Design review of the part built by this model. Coordinates are the model's own, in mm. A direction names the side the tool comes from. Round coordinates to 2 decimals unless told otherwise and drop trailing zeros. Order: outer loops, then holes, each group sorted by start corner. A loop starts at its lowest first (then second) coordinate and runs counter-clockwise, first axis right, second up. Notation, with made-up numbers: (7, -21) - (16, -21) arc R12 ccw to (16, -2) - close; hole circle Ø10 at (54.5, 77). An arc over 180 degrees is marked (long way). Answer as a JSON object with one key per item and string values. Group by question number.
from build123d import *

# Parameters (mm, degrees)
EXTRUDE_1_DEPTH     = 50
SKETCH_2_W          = 4
SKETCH_2_H          = 24
EXTRUDE_2_DEPTH     = 210
CUT_EXTRUDE_1_DEPTH = 93
SKETCH_4_W          = 4
SKETCH_4_H          = 24
EXTRUDE_3_DEPTH     = 260
EXTRUDE_4_DEPTH     = 30
SKETCH_6_R          = 4
CUT_EXTRUDE_2_DEPTH = 97
SKETCH_8_W          = 162.90282803
SKETCH_8_H          = 303.086270548
CUT_EXTRUDE_4_DEPTH = 86
EXTRUDE_5_DEPTH     = 40
SKETCH_10_R         = 10
EXTRUDE_6_DEPTH     = 80


with BuildPart() as part:
    # 草图1 → 凸台-拉伸1 (new body, symmetric)
    with BuildSketch(Plane(origin=(0, 0, 0), x_dir=(1, 0, 0), z_dir=(0, 1, 0))):
        with BuildLine():
            Line((-46, 0), (-46, 12))
            Line((-46, 12), (-42, 12))
            Line((-42, 12), (-42, 0))
            ThreePointArc((-42, 0), (0, -42), (42, 0))
            Line((42, 0), (42, 12))
            Line((42, 12), (46, 12))
            Line((46, 12), (46, 0))
            ThreePointArc((46, 0), (37.456641601, -26.702059846), (15, -43.48562981))
            Line((15, -43.48562981), (15, -73))
            Line((15, -73), (10, -73))
            Line((10, -73), (10, -53))
            Line((10, -53), (-10, -53))
            Line((-10, -53), (-10, -73))
            Line((-10, -73), (-15, -73))
            Line((-15, -73), (-15, -43.48562981))
            ThreePointArc((-15, -43.48562981), (-37.456641601, -26.702059846), (-46, 0))
        make_face()
    extrude(amount=EXTRUDE_1_DEPTH, both=True)

    # 草图2 → 凸台-拉伸2 (add)
    with BuildSketch(Plane(origin=(0, 50, 0), x_dir=(1, 0, 0), z_dir=(0, 1, 0))):
        with Locations((-44, 0)):
            Rectangle(SKETCH_2_W, SKETCH_2_H)
        with Locations((44, 0)):
            Rectangle(SKETCH_2_W, SKETCH_2_H)
    extrude(amount=-EXTRUDE_2_DEPTH)

    # 草图3 → 切除-拉伸1 (cut, through all)
    with BuildSketch(Plane(origin=(46, 0, 0), x_dir=(0, 0, -1), z_dir=(1, 0, 0))):
        with BuildLine():
            Line((-12, -138), (-12, -169.379550042))
            Line((-12, -169.379550042), (12, -169.379550042))
            Line((12, -169.379550042), (12, -138))
            ThreePointArc((12, -138), (0, -150), (-12, -138))
        make_face()
    extrude(amount=-CUT_EXTRUDE_1_DEPTH, mode=Mode.SUBTRACT)

    # 草图4 → 凸台-拉伸3 (add)
    with BuildSketch(Plane(origin=(0, 50, 0), x_dir=(1, 0, 0), z_dir=(0, 1, 0))):
        with Locations((44, 0)):
            Rectangle(SKETCH_4_W, SKETCH_4_H)
        with Locations((-44, 0)):
            Rectangle(SKETCH_4_W, SKETCH_4_H)
    extrude(amount=EXTRUDE_3_DEPTH)

    # 草图5 → 凸台-拉伸4 (add)
    with BuildSketch(Plane(origin=(0, 310, 0), x_dir=(1, 0, 0), z_dir=(0, 1, 0))):
        with BuildLine():
            Line((-48.538644398, 12), (-42, 12))
            Line((-42, 12), (-42, 0))
            ThreePointArc((-42, 0), (0, -42), (42, 0))
            Line((42, 0), (42, 12))
            Line((42, 12), (48.538644398, 12))
            ThreePointArc((48.538644398, 12), (0, -50), (-48.538644398, 12))
        make_face()
    extrude(amount=-EXTRUDE_4_DEPTH)

    # 草图6 → 切除-拉伸2 (cut, through all)
    with BuildSketch(Plane(origin=(46, 0, 0), x_dir=(0, 0, -1), z_dir=(1, 0, 0))):
        with Locations((0, 200)):
            Circle(SKETCH_6_R)
    extrude(amount=-CUT_EXTRUDE_2_DEPTH, mode=Mode.SUBTRACT)

    # 草图8 → 切除-拉伸4 (cut, through all)
    with BuildSketch(Plane(origin=(0, 0, -12), x_dir=(-1, 0, 0), z_dir=(0, 0, -1))):
        with Locations((10.670277924, 166.543135274)):
            Rectangle(SKETCH_8_W, SKETCH_8_H)
    extrude(amount=-CUT_EXTRUDE_4_DEPTH, mode=Mode.SUBTRACT)

    # 草图9 → 凸台-拉伸5 (add)
    with BuildSketch(Plane.XZ.offset(50)):
        with BuildLine():
            Line((-50, 0), (-46, 0))
            ThreePointArc((-46, 0), (0, 46), (46, 0))
            Line((46, 0), (50, 0))
            ThreePointArc((50, 0), (0, 50), (-50, 0))
        make_face()
    extrude(amount=-EXTRUDE_5_DEPTH)

    # 草图10 → 凸台-拉伸6 (add, symmetric)
    with BuildSketch(Plane(origin=(0, 0, 0), x_dir=(0, 0, -1), z_dir=(1, 0, 0))):
        with Locations((-60.348480035, -40)):
            Circle(SKETCH_10_R)
    extrude(amount=EXTRUDE_6_DEPTH, both=True)


solid = part.part
1. Tool access review of faces 4 (the cylindrical face through (-33.4, 2.68, 31.63)), 5 (the cylindrical face through (-40, -30, 30)), 6 (the cylindrical face through (-47.04, -48.87, 55.73)), 7 (the cylindrical face through (40.572, -30.28, 29.222)), 8 (the flat face through (44, -95, 12)): name each direction out of +Z, -Z, +X, -X, +Y, -Y from which nothing blocks a thin tool from reaching the whole face with its end or side.
2. Take a section at B-B, the plane z = 5.5. Give the boundary of the cut face in (x, y).
3. Mouldability with a two-part tool opening along X and no side actions: class faces 1 (the cylindrical face through (44, -150, 0)), 2 (the flat face through (-46, -69, 0)), 3 (the cylindrical face through (0.14, -39.665, 70.343)) as pulls with the +X half, pulls with the -X half, needs draft (parallel to the pull), parting line crosses it, or undercut.
4. Take a section at C-C, the plane x = 21. Give the boundary of the cut face in (y, z).
5. Clearance check with flat-ended pins moving along their axes: P1, Ø19, axis at y = -26.5, z = -5, coming from the +X side; P2, Ø12, axis at y = -67.5, z = 0, coming from the -X side; P3, Ø8, axis at x = 18.5, y = -21, coming from the -Z side; P4, Ø8, axis at y = -93, z = 19, coming from the -X side. State where each tip first meets the part, or that it passes through.
6. Take a section at D-D, the plane y = -40. Give the boundary of the cut face in (x, z).
7. Take a section at A-A, the plane y = -110. Give the boundary of the cut face in (x, z).
8. To check wall thickness, follow line 1 (X direction, y = -7, z = 64); line 2 (X direction, y = -79.5, z = -2.5); line 3 (Z direction, x = -17.5, y = -45.5). State the ranges of each line that lie inside material, in increasing order. Write a range as from..to.
Response values:
{
 "1": {"face 4": "+Z, -X, +Y", "face 5": "-X, +Y, -Y", "face 6": "-X", "face 7": "+X, +Y, -Y", "face 8": "+Z, +X, -X, -Y"},
 "2": {"outline": "(-49.7, -50) - (-46, -50) - (-46, -148.67) - (-42, -148.67) - (-42, -50) - (-41.64, -50) - (-41.64, 15) - (-46, 15) - (-46, -10) - (-49.7, -10) - close; (41.64, -50) - (42, -50) - (42, -148.67) - (46, -148.67) - (46, -50) - (49.7, -50) - (49.7, -10) - (46, -10) - (46, 15) - (41.64, 15) - close"},
 "3": {"face 1": "needs draft", "face 2": "pulls with the -X half", "face 3": "undercut"},
 "4": {"outline": "(-50, 36.37) - (15, 36.37) - (15, 40.93) - (-10, 40.93) - (-10, 45.38) - (-50, 45.38) - close; circle Ø20 at (-40, 60.35)"},
 "5": {"P1": "x = 50", "P2": "x = -46", "P3": "z = 35.46", "P4": "through"},
 "6": {"outline": "(-80, 50.35) - (-15, 50.35) - (-15, 47.7) arc R50 ccw to (-50, 0) - (-46, 0) - (-46, -12) - (-42, -12) - (-42, 0) arc R42 cw to (42, 0) - (42, -12) - (46, -12) - (46, 0) - (50, 0) arc R50 ccw to (15, 47.7) - (15, 50.35) - (80, 50.35) - (80, 70.35) - (15, 70.35) - (15, 73) - (10, 73) - (10, 70.35) - (-10, 70.35) - (-10, 73) - (-15, 73) - (-15, 70.35) - (-80, 70.35) - close"},
 "7": {"outline": "(-46, -12) - (-42, -12) - (-42, 12) - (-46, 12) - close; (42, -12) - (46, -12) - (46, 12) - (42, 12) - close"},
 "8": {"line 1": "-15..-10, 10..15", "line 2": "-46..-42, 42..46", "line 3": "38.18..46.84, 52..68.7"}
}
